```python
from build123d import *

# Parameters (mm, degrees)
BOSS_EXTRUDE1_DEPTH     = 40
FILLET1_R               = 10
CUT_EXTRUDE1_DEPTH      = 30
SKETCH4_R               = 10
BOSS_EXTRUDE3_DEPTH     = 10
CUT_EXTRUDE2_REACH      = 181.038
CUT_EXTRUDE2_END_RADIUS = 60
SKETCH5_W               = 20
SKETCH5_H               = 40
FILLET2_R               = 5
CUT_EXTRUDE3_REACH      = 153.142
SKETCH6_R               = 1
SKETCH7_R               = 2.5
CUT_EXTRUDE4_DEPTH      = 5
CUT_EXTRUDE5_REACH      = 149.119
SKETCH8_R               = 0.8
SKETCH9_R               = 3
CUT_EXTRUDE6_DEPTH      = 10
SKETCH11_R              = 5
CUT_EXTRUDE7_DEPTH      = 3
SKETCH12_R              = 6
CUT_EXTRUDE8_DEPTH      = 20
FILLET3_R               = 15


with BuildPart() as part:
    # Sketch1 → Boss-Extrude1 (new body)
    with BuildSketch(Plane(origin=(0, 0, 0), x_dir=(1, 0, 0), z_dir=(0, 1, 0))):
        with BuildLine():
            Line((-67.694698117, 31.515169882), (112.305301883, 31.515169882))
            ThreePointArc((112.305301883, 31.515169882), (142.305301883, 1.515169882), (112.305301883, -28.484830118))
            Line((112.305301883, -28.484830118), (-67.694698117, -28.484830118))
            ThreePointArc((-67.694698117, -28.484830118), (-97.694698117, 1.515169882), (-67.694698117, 31.515169882))
        make_face()
    extrude(amount=BOSS_EXTRUDE1_DEPTH)

    # Fillet1
    fillet1_edges = [part.edges().sort_by_distance(p)[0] for p in [
        (142.305301883, 40, -1.515169882),
        (22.305301883, 40, -31.515169882),
        (-97.694698117, 40, -1.515169882),
        (22.305301883, 40, 28.484830118),
    ]]
    fillet(fillet1_edges, radius=FILLET1_R)

    # Sketch3 → Cut-Extrude1 (cut)
    with BuildSketch(Plane.XZ):
        with BuildLine():
            Line((73.949041486, -31.515169882), (148.949041486, -31.515169882))
            Line((148.949041486, -31.515169882), (148.949041486, 28.484830118))
            Line((148.949041486, 28.484830118), (73.949041486, 28.484830118))
            ThreePointArc((73.949041486, 28.484830118), (65.910565713, -1.515169882), (73.949041486, -31.515169882))
        make_face()
        with BuildLine():
            Line((-29.33843772, 28.484830118), (-104.33843772, 28.484830118))
            Line((-104.33843772, 28.484830118), (-104.33843772, -31.515169882))
            Line((-104.33843772, -31.515169882), (-29.33843772, -31.515169882))
            ThreePointArc((-29.33843772, -31.515169882), (-21.299961947, -1.515169882), (-29.33843772, 28.484830118))
        make_face()
    extrude(amount=-CUT_EXTRUDE1_DEPTH, mode=Mode.SUBTRACT)

    # Sketch4 → Boss-Extrude3 (add)
    with BuildSketch(Plane(origin=(0, 30, 0), x_dir=(-1, 0, 0), z_dir=(0, -1, 0))):
        with Locations(Location((-112.305301883, 1.515169882, 0), (0, 0, 90))):
            Circle(SKETCH4_R)
        with Locations(Location((67.694698117, 1.515169882, 0), (0, 0, 270))):
            Circle(SKETCH4_R)
    extrude(amount=BOSS_EXTRUDE3_DEPTH)

    # Cut-Extrude2: up to this cylinder (the profile starts outside it)
    cut_extrude2_end = Plane(origin=(-81.299961947, 0, -1.515169882), z_dir=(0, -1, 0)) * Cylinder(CUT_EXTRUDE2_END_RADIUS, 483.076, mode=Mode.PRIVATE)
    # Sketch5 → Cut-Extrude2 (cut, up to the surface)
    with BuildSketch(Plane(origin=(73.949041486, 0, 0), x_dir=(0, 0, -1), z_dir=(1, 0, 0)), mode=Mode.PRIVATE) as cut_extrude2_sk1:
        with Locations((1.515169882, 0)):
            Rectangle(SKETCH5_W, SKETCH5_H)
    cut_extrude2_tool1 = extrude(cut_extrude2_sk1.sketch, amount=-CUT_EXTRUDE2_REACH, mode=Mode.PRIVATE) - cut_extrude2_end
    add(cut_extrude2_tool1.solids().sort_by_distance((73.949041, 0, -1.51517))[0], mode=Mode.SUBTRACT)

    # Fillet2
    # the kernel refuses this fillet: 5 mm, written as the material it takes off along each edge
    with BuildSketch(Plane(origin=(-29.33843772, -20.096189432, 28.484830118), x_dir=(0.44322659401027775, 0, -0.8964096085841831), z_dir=(0, 1, 0))) as fillet2_piece_1:
        with BuildLine():
            CenterArc((8.044914281, -4.989633951), FILLET2_R, 93.690067526, 112.619864948)
            Line((3.562866238, -7.205766921), (0, 0))
            ThreePointArc((0, 0), (3.861558855, -0.124392586), (7.72311771, 0))
        make_face()
    extrude(amount=50.096189432, mode=Mode.SUBTRACT)
    with BuildSketch(Plane(origin=(-29.33843772, -20.096189432, -31.515169882), x_dir=(1, 0, 0), z_dir=(0, 1, 0))) as fillet2_piece_2:
        with BuildLine():
            CenterArc((8.038475773, -5), FILLET2_R, 90, 112.619864948)
            ThreePointArc((3.423091158, -6.923076923), (1.823052288, -3.406404359), (0, 0))
            Line((0, 0), (8.038475773, 0))
        make_face()
    extrude(amount=50.096189432, mode=Mode.SUBTRACT)
    with BuildSketch(Plane(origin=(73.949041486, -20.096189432, -31.515169882), x_dir=(-1, 0, 0), z_dir=(0, 1, 0))) as fillet2_piece_3:
        with BuildLine():
            CenterArc((8.038475773, 5), FILLET2_R, 157.380135052, 112.619864948)
            ThreePointArc((3.423091158, 6.923076923), (1.823052288, 3.406404359), (0, 0))
            Line((0, 0), (8.038475773, 0))
        make_face()
    extrude(amount=50.096189432, mode=Mode.SUBTRACT)
    with BuildSketch(Plane(origin=(73.949041486, -20.096189432, 28.484830118), x_dir=(-0.4432265940102763, 0, -0.8964096085841838), z_dir=(0, 1, 0))) as fillet2_piece_4:
        with BuildLine():
            CenterArc((8.044914281, 4.989633951), FILLET2_R, 153.690067526, 112.619864948)
            Line((3.562866238, 7.205766921), (0, 0))
            ThreePointArc((0, 0), (3.861558855, 0.124392586), (7.72311771, 0))
        make_face()
    extrude(amount=50.096189432, mode=Mode.SUBTRACT)

    # Sketch6 → Cut-Extrude3 (cut, up to next)
    with BuildSketch(Plane(origin=(0, 0, 0), x_dir=(-1, 0, 0), z_dir=(0, -1, 0)), mode=Mode.PRIVATE) as cut_extrude3_sk1:
        with Locations(Location((10.194698117, -15.984830118, 0), (0, 0, 90))):
            Circle(SKETCH6_R)
    cut_extrude3_tool1 = extrude(cut_extrude3_sk1.sketch, amount=-CUT_EXTRUDE3_REACH, mode=Mode.PRIVATE) & part.part
    # Sketch6 → Cut-Extrude3 (cut, up to next)
    with BuildSketch(Plane(origin=(0, 0, 0), x_dir=(-1, 0, 0), z_dir=(0, -1, 0)), mode=Mode.PRIVATE) as cut_extrude3_sk2:
        with Locations(Location((-54.805301883, -15.984830118, 0), (0, 0, 90))):
            Circle(SKETCH6_R)
    cut_extrude3_tool2 = extrude(cut_extrude3_sk2.sketch, amount=-CUT_EXTRUDE3_REACH, mode=Mode.PRIVATE) & part.part
    # Sketch6 → Cut-Extrude3 (cut, up to next)
    with BuildSketch(Plane(origin=(0, 0, 0), x_dir=(-1, 0, 0), z_dir=(0, -1, 0)), mode=Mode.PRIVATE) as cut_extrude3_sk3:
        with Locations(Location((-54.805301883, 19.015169882, 0), (0, 0, 90))):
            Circle(SKETCH6_R)
    cut_extrude3_tool3 = extrude(cut_extrude3_sk3.sketch, amount=-CUT_EXTRUDE3_REACH, mode=Mode.PRIVATE) & part.part
    # Sketch6 → Cut-Extrude3 (cut, up to next)
    with BuildSketch(Plane(origin=(0, 0, 0), x_dir=(-1, 0, 0), z_dir=(0, -1, 0)), mode=Mode.PRIVATE) as cut_extrude3_sk4:
        with Locations(Location((10.194698117, 19.015169882, 0), (0, 0, 90))):
            Circle(SKETCH6_R)
    cut_extrude3_tool4 = extrude(cut_extrude3_sk4.sketch, amount=-CUT_EXTRUDE3_REACH, mode=Mode.PRIVATE) & part.part
    add(cut_extrude3_tool1.solids().sort_by_distance((-10.194698, 0, 15.98483))[0], mode=Mode.SUBTRACT)
    add(cut_extrude3_tool2.solids().sort_by_distance((54.805302, 0, 15.98483))[0], mode=Mode.SUBTRACT)
    add(cut_extrude3_tool3.solids().sort_by_distance((54.805302, 0, -19.01517))[0], mode=Mode.SUBTRACT)
    add(cut_extrude3_tool4.solids().sort_by_distance((-10.194698, 0, -19.01517))[0], mode=Mode.SUBTRACT)

    # Sketch7 → Cut-Extrude4 (cut)
    with BuildSketch(Plane(origin=(0, 40, 0), x_dir=(1, 0, 0), z_dir=(0, 1, 0))):
        with Locations(Location((-10.194698117, 19.015169882, 0), (0, 0, 270))):
            Circle(SKETCH7_R)
        with Locations(Location((-10.194698117, -15.984830118, 0), (0, 0, 270))):
            Circle(SKETCH7_R)
        with Locations(Location((54.805301883, -15.984830118, 0), (0, 0, 270))):
            Circle(SKETCH7_R)
        with Locations(Location((54.805301883, 19.015169882, 0), (0, 0, 270))):
            Circle(SKETCH7_R)
    extrude(amount=-CUT_EXTRUDE4_DEPTH, mode=Mode.SUBTRACT)

    # Sketch8 → Cut-Extrude5 (cut, up to next)
    with BuildSketch(Plane(origin=(0, 20, 0), x_dir=(-1, 0, 0), z_dir=(0, -1, 0)), mode=Mode.PRIVATE) as cut_extrude5_sk1:
        with Locations(Location((67.694698117, 1.515169882, 0), (0, 0, 90))):
            Circle(SKETCH8_R)
    cut_extrude5_tool1 = extrude(cut_extrude5_sk1.sketch, amount=-CUT_EXTRUDE5_REACH, mode=Mode.PRIVATE) & part.part
    # Sketch8 → Cut-Extrude5 (cut, up to next)
    with BuildSketch(Plane(origin=(0, 20, 0), x_dir=(-1, 0, 0), z_dir=(0, -1, 0)), mode=Mode.PRIVATE) as cut_extrude5_sk2:
        with Locations(Location((-112.305301883, 1.515169882, 0), (0, 0, 90))):
            Circle(SKETCH8_R)
    cut_extrude5_tool2 = extrude(cut_extrude5_sk2.sketch, amount=-CUT_EXTRUDE5_REACH, mode=Mode.PRIVATE) & part.part
    add(cut_extrude5_tool1.solids().sort_by_distance((-67.694698, 20, -1.51517))[0], mode=Mode.SUBTRACT)
    add(cut_extrude5_tool2.solids().sort_by_distance((112.305302, 20, -1.51517))[0], mode=Mode.SUBTRACT)

    # Sketch9 → Cut-Extrude6 (cut)
    with BuildSketch(Plane(origin=(0, 20, 0), x_dir=(-1, 0, 0), z_dir=(0, -1, 0))):
        with Locations(Location((67.694698117, 1.515169882, 0), (0, 0, 90))):
            Circle(SKETCH9_R)
        with Locations(Location((-112.305301883, 1.515169882, 0), (0, 0, 90))):
            Circle(SKETCH9_R)
    extrude(amount=-CUT_EXTRUDE6_DEPTH, mode=Mode.SUBTRACT)

    # Sketch11 → Cut-Extrude7 (cut)
    with BuildSketch(Plane(origin=(0, 40, 0), x_dir=(1, 0, 0), z_dir=(0, 1, 0))):
        with Locations(Location((-67.694698117, 1.515169882, 0), (0, 0, 270))):
            Circle(SKETCH11_R)
        with Locations(Location((112.305301883, 1.515169882, 0), (0, 0, 270))):
            Circle(SKETCH11_R)
    extrude(amount=-CUT_EXTRUDE7_DEPTH, mode=Mode.SUBTRACT)

    # Sketch12 → Cut-Extrude8 (cut)
    with BuildSketch(Plane(origin=(0, 0, 0), x_dir=(-1, 0, 0), z_dir=(0, -1, 0))):
        with Locations((22.139164116, -8.484830118)):
            Circle(SKETCH12_R)
        with Locations((22.139164116, 11.515169882)):
            Circle(SKETCH12_R)
        with Locations((-66.749767882, 11.515169882)):
            Circle(SKETCH12_R)
        with Locations((-66.749767882, -8.484830118)):
            Circle(SKETCH12_R)
    extrude(amount=-CUT_EXTRUDE8_DEPTH, mode=Mode.SUBTRACT)

    # Fillet3
    fillet3_edges = [part.edges().sort_by_distance(p)[0] for p in [
        (68.044321089, 10, 14.343510174),
        (60.749767882, 10, 8.484830118),
        (68.044321089, 10, -17.373849938),
        (60.749767882, 10, -11.515169882),
        (-23.433717323, 10, -17.373849938),
        (-16.139164116, 10, -11.515169882),
        (-23.433717323, 10, 14.343510174),
        (-16.139164116, 10, 8.484830118),
    ]]
    fillet(fillet3_edges, radius=FILLET3_R)


solid = part.part
```
The listing builds one solid part. Answer for the finished solid, in the listing's coordinates (mm). A direction names the side the tool comes from. Coordinates: 2 decimals unless noted, no trailing zeros. Loops run counter-clockwise (first coordinate to the right, second up) from the corner with the lowest first, then second, coordinate; pieces in that order, holes last. Notation, with made-up numbers: (31, -12.5) - (89, -12.5) arc R23 ccw to (89, 1.5) - close; hole circle Ø8 at (0.5, 41). An arc over 180 degrees is marked (long way). Use a Markdown table: item, result. Add a question column.
1) The mould has two halves that part along X. Classify faces 1 (the flat face through (95, 30, -1)), 2 (the flat face through (23, 20, -2)), 3 (the cylindrical face through (-13.04, 9.86, -12.6)): released by +X, released by -X, zero draft, split by the parting line, or undercut.
2) Given pin 1 (3 mm diameter, centred on x = 71.5, z = 12, fed in from -Y); pin 2 (3 mm diameter, centred on x = -69.5, z = -3, fed in from +Y); pin 3 (1 mm diameter, centred on y = 32, z = 14.5, fed in from +X), each flat-ended and moving along its own axis, determine where each tip first touches the part or whether it passes through.
3) The part is cut by section A-A, the plane y = 25. State how many separate pieces and enclosed holes the cut face has, and give its area (3 significant figures).
4) The part is cut by section C-C, the plane x = -28.5. Give the vertices of the cut face in (y, z).
5) For faces 4 (the cylindrical face through (-62.737, 38.521, -2.166)), 5 (the cylindrical face through (57.65, 10.14, -12.6)), 6 (the cylindrical face through (102.543, 25.07, 0.653)), determine the directions among +Z, -Z, +X, -X, +Y, -Y from which every point of the face is accessible in a straight line to the end or side of a thin tool.
6) Find the intervals of material crossed by line 1 (X direction, y = 12.5, z = -19); line 2 (Z direction, x = 42, y = 10.5); line 3 (Z direction, x = 55, y = 8.5), in increasing order.
Here are the results:
| question | item | result |
|---|---|---|
| 1 | face 1 | undercut |
| 1 | face 2 | zero draft |
| 1 | face 3 | released by -X |
| 2 | pin 1 | stops at y = 30 |
| 2 | pin 2 | stops at y = 37 |
| 2 | pin 3 | stops at x = 137.77 |
| 3 | separate pieces | 3 |
| 3 | enclosed holes | 6 |
| 3 | area | 6,050 mm^2 |
| 4 | outline | (30, -31.52) arc R10 ccw to (40, -21.52) - (40, 18.48) arc R10 ccw to (30, 28.48) - close |
| 5 | face 4 | +Y |
| 5 | face 5 | +X, -Y |
| 5 | face 6 | -Y |
| 6 | line 1 | x = -22.24 to -11.19, -9.19 to 53.81, 55.81 to 66.85 |
| 6 | line 2 | z = -31.52 to -11.52, 8.48 to 28.48 |
| 6 | line 3 | z = -31.52 to -20, -18.03 to -11.81, 8.78 to 15, 16.97 to 28.48 |
